```python
from build123d import *

# Parameters (mm, degrees)
SKETCH3_R          = 9.525
BASE_EXTRUDE_DEPTH = 19.05
SKETCH4_R          = 12.7
CUT_EXTRUDE1_DEPTH = 38.1


with BuildPart() as part:
    # Sketch3 → Base-Extrude (new, symmetric)
    with BuildSketch(Plane.XY):
        with BuildLine():
            Line((-69.85, 25.4), (0, 25.4))
            Line((0, 25.4), (0, -25.4))
            Line((0, -25.4), (-69.85, -25.4))
            ThreePointArc((-69.85, -25.4), (-95.25, 0), (-69.85, 25.4))
        make_face()
        with Locations(Location((-69.85, 0, 0), (0, 0, 180))):
            Circle(SKETCH3_R, mode=Mode.SUBTRACT)
    extrude(amount=BASE_EXTRUDE_DEPTH, both=True)

    # Sketch4 → Cut-Extrude1 (cut)
    with BuildSketch(Plane(origin=(0, 0, 0), x_dir=(0, 0, -1), z_dir=(1, 0, 0))):
        with Locations(Location((0, 0, 0), (0, 0, 90))):
            Circle(SKETCH4_R)
    extrude(amount=-CUT_EXTRUDE1_DEPTH, mode=Mode.SUBTRACT)


solid = part.part
```
Could you check a few things on this model? Use its own coordinates, in mm. A direction names the side the tool comes from. Coordinates: 2 decimals unless noted, no trailing zeros. Write each loop counter-clockwise with the first axis right and the second up, starting at its lowest first coordinate (ties: lowest second). Pieces come first, ordered by that corner, then holes. Notation, with made-up numbers: M -38.5,22 L 9.5,22 A30 cw 9.5,48 Z; hole C 82.25,44.5 d4. An arc over 180 degrees is marked long. Answer as CSV lines item,"result". Start each with the question number.
1) For P1, Ø10, axis at y = 7.5, z = 0, coming from the +X side; P2, Ø1, axis at y = 6.5, z = -9, coming from the -X side, each with a flat end and sliding along its axis, tell me the tip position at first contact or that it passes through.
2) For faces 4 (the flat face through (-47, 0, -19.05)), 5 (the cylindrical face through (-18.8, -10.1, -7.7)), which set-ups out of +Z, -Z, +X, -X, +Y, -Y let a thin tool reach every point of the face, with its end or its side?
3) I want a section at C-C, the plane x = -77.5. Please give me the cut outline in (y, z).
4) Please list where these lines run through material, in increasing order: line 1 (Z direction, x = -16, y = 0); line 2 (Y direction, x = -69.85, z = -10) (3 decimals); line 3 (X direction, y = 8, z = -3). Write a range as from..to.
5) I want a section at D-D, the plane x = -26. Please give me the cut outline in (y, z).
6) I want a section at B-B, the plane y = 0. Please give me the cut outline in (x, z) (3 decimals), and give its area (3 significant figures).
7) I want a section at A-A, the plane z = 0. Please give me the cut outline in (x, y) (3 decimals), and give its area (3 significant figures).
8) We'd pull the mould along Y, two halves only. Please class faces 1 (the flat face through (0, 0, 13)), 2 (the cylindrical face through (-95.244, -0.559, 0.267)), 3 (the flat face through (-38.1, 0, 0)): +Y half, -Y half, draft (parallel to the pull), parting line (faces both ways), or undercut.
Data:
1,P1,"stops at x = -38.1"
1,P2,"stops at x = -94.53"
2,face 4,"-Z, +X, -X, +Y, -Y"
2,face 5,"+X"
3,outline,"M -24.22,-19.05 L -5.67,-19.05 L -5.67,19.05 L -24.22,19.05 Z; M 5.67,-19.05 L 24.22,-19.05 L 24.22,19.05 L 5.67,19.05 Z"
4,line 1,"z = -19.05..-12.7, 12.7..19.05"
4,line 2,"y = -25.4..-9.525, 9.525..25.4"
4,line 3,"x = -93.96..-75.02, -64.68..-38.1"
5,outline,"M -25.4,-19.05 L 25.4,-19.05 L 25.4,19.05 L -25.4,19.05 Z; hole C 0,0 d25.4"
6,outline,"M -95.25,-19.05 L -79.375,-19.05 L -79.375,19.05 L -95.25,19.05 Z; M -60.325,-19.05 L 0,-19.05 L 0,-12.7 L -38.1,-12.7 L -38.1,12.7 L 0,12.7 L 0,19.05 L -60.325,19.05 Z"
6,area,"1,940 mm^2"
7,outline,"M -69.85,-25.4 L 0,-25.4 L 0,-12.7 L -38.1,-12.7 L -38.1,12.7 L 0,12.7 L 0,25.4 L -69.85,25.4 A25.4 ccw Z; hole C -69.85,0 d19.05"
7,area,"3,310 mm^2"
8,face 1,"draft"
8,face 2,"parting line"
8,face 3,"undercut"
